Verification items for the finished model (mm, model axes). Face numbers are marked on the shaded views. A direction names the side the tool comes from. Round coordinates to 2 decimals unless told otherwise and drop trailing zeros. Order: outer loops, then holes, each group sorted by start corner. A loop starts at its lowest first (then second) coordinate and runs counter-clockwise, first axis right, second up. Notation, with made-up numbers: (-23.75, -10.75) -> (-2.75, -10.75) arc R23 ccw to (-2.75, 7.25) -> close; hole circle Ø10 at (70, 35). An arc over 180 degrees is marked (long way). Return JSON: item names as keys, results as strings. Group by question number.
1) Scan lines: L1, parallel to Z at x = 0.5, y = -47; L2, parallel to Y at x = -0.5, z = 18; L3, parallel to X at y = -21, z = 2.5. Record each from-to range of solid material in increasing order.
2) Depth check by flat-ended pin: pin 1 (5 mm diameter, centred on x = -1.5, y = -27.5, fed in from +Z); pin 2 (5.5 mm diameter, centred on x = 20.44, y = -14.74, fed in from -Z); pin 3 (8 mm diameter, centred on x = 18, z = -14.5, fed in from -Y); pin 4 (3 mm diameter, centred on x = -11.5, z = -6, fed in from +Y). Enter the tip coordinate at first touch or a pass-through.
3) Draft check along X on the marked faces 1, 2 and 3. Enter one of: pulls with the +X half, pulls with the -X half, needs draft (parallel to the pull), parting line crosses it, or undercut.
4) Tool access check on the marked faces 4, 5, 6, 7 and 8. Record the directions out of +Z, -Z, +X, -X, +Y, -Y that give a thin tool (end or side, any length) a straight path to the whole face; none if there is none.
5) Section check D-D on z = -16. Enter the section's corners in (x, y), plus the area to 3 significant figures.
6) Section check A-A on z = 14. Enter the section's corners in (x, y).
7) Section check B-B on x = -17.5. Enter the section's corners in (y, z), plus the area to 3 significant figures.
8) Section check C-C on y = -36. Enter the section's corners in (x, z).
```python
from build123d import *

# Parameters (mm, degrees)
F0_R     = 3
F1_DEPTH = 3
F2_W     = 60
F2_H     = 40
F2_R     = 3.5
F3_DEPTH = 3


with BuildPart() as f1:
    # F0 (on Top) → F1 (new body, symmetric)
    with BuildSketch(Plane.XY):
        with BuildLine():
            ThreePointArc((18.440057, -7.743663), (9.577003, -17.557933), (-3.472964, -19.696155))
            Line((-3.472964, -19.696155), (-31.559943, -14.743663))
            Line((-31.559943, -14.743663), (-31.559943, -47.743663))
            Line((-31.559943, -47.743663), (28.440057, -47.743663))
            Line((28.440057, -47.743663), (28.440057, -10.743663))
            ThreePointArc((28.440057, -10.743663), (27.561377, -8.622342), (25.440057, -7.743663))
            Line((25.440057, -7.743663), (18.440057, -7.743663))
        make_face()
        with Locations((-23.559943, -22.743663)):
            Circle(F0_R, mode=Mode.SUBTRACT)
        with Locations((20.440057, -14.743663)):
            Circle(F0_R, mode=Mode.SUBTRACT)
    extrude(amount=F1_DEPTH, both=True)

    # F2 (on face) → F3 (join)
    with BuildSketch(Plane.XZ.offset(47.743663)):
        with Locations((-1.559943, 0)):
            Rectangle(F2_W, F2_H)
        with Locations((-23.559943, -14)):
            Circle(F2_R, mode=Mode.SUBTRACT)
        with Locations((20.440057, -14)):
            Circle(F2_R, mode=Mode.SUBTRACT)
        with Locations((-23.559943, 14)):
            Circle(F2_R, mode=Mode.SUBTRACT)
        with Locations((20.440057, 14)):
            Circle(F2_R, mode=Mode.SUBTRACT)
    extrude(amount=F3_DEPTH)


solid = f1.part
```
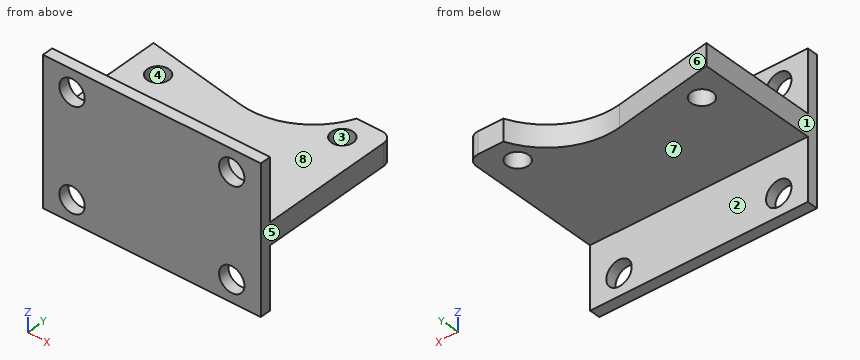
Check result:
{
 "1": {"L1": "-3 to 3", "L2": "-50.74 to -47.74", "L3": "-31.56 to -26, -21.12 to 28.44"},
 "2": {"pin 1": "z = 3", "pin 2": "through", "pin 3": "y = -50.74", "pin 4": "y = -47.74"},
 "3": {"face 1": "pulls with the -X half", "face 2": "needs draft", "face 3": "undercut"},
 "4": {"face 4": "+Z, -Z", "face 5": "+Z, -Z, +X, +Y, -Y", "face 6": "+Z, -Z, +Y", "face 7": "-Z, +X, -X, +Y", "face 8": "+Z, +X, -X, +Y"},
 "5": {"outline": "(-31.56, -50.74) -> (-26.43, -50.74) -> (-26.43, -47.74) -> (-31.56, -47.74) -> close; (-20.69, -50.74) -> (17.57, -50.74) -> (17.57, -47.74) -> (-20.69, -47.74) -> close; (23.31, -50.74) -> (28.44, -50.74) -> (28.44, -47.74) -> (23.31, -47.74) -> close", "area": "146 mm^2"},
 "6": {"outline": "(-31.56, -50.74) -> (-27.06, -50.74) -> (-27.06, -47.74) -> (-31.56, -47.74) -> close; (-20.06, -50.74) -> (16.94, -50.74) -> (16.94, -47.74) -> (-20.06, -47.74) -> close; (23.94, -50.74) -> (28.44, -50.74) -> (28.44, -47.74) -> (23.94, -47.74) -> close"},
 "7": {"outline": "(-50.74, -20) -> (-47.74, -20) -> (-47.74, -3) -> (-17.22, -3) -> (-17.22, 3) -> (-47.74, 3) -> (-47.74, 20) -> (-50.74, 20) -> close", "area": "303 mm^2"},
 "8": {"outline": "(-31.56, -3) -> (28.44, -3) -> (28.44, 3) -> (-31.56, 3) -> close"}
}
